```python
from build123d import *

# Parameters (mm, degrees)
F0_R      = 15.24
F0_R_2    = 11.43
F1_DEPTH  = 2.9972
F3_DEPTH  = 26.67
F4_R      = 15.24
F4_R_2    = 11.43
F5_DEPTH  = 2.54
F6_W      = 9.144
F6_H      = 6.35
F7_DEPTH  = 28.575
F8_W      = 1.27
F8_H      = 6.096
F9_DEPTH  = 2.54
F10_R     = 24.638
F10_R_2   = 15.24
F11_DEPTH = 3.81
F12_DEPTH = 11.43
F13_R     = 15.24
F13_R_2   = 11.43
F14_DEPTH = 20.955
F16_DEPTH = 3.4544
F17_R     = 15.24
F17_R_2   = 11.43
F18_DEPTH = 3.175
F19_DEPTH = 25.4
F20_R     = 1.5621
F21_DEPTH = 6.35


with BuildPart() as f1:
    # F0 (on Front) → F1 (new body)
    with BuildSketch(Plane.XZ):
        Circle(F0_R)
        Circle(F0_R_2, mode=Mode.SUBTRACT)
    extrude(amount=F1_DEPTH)

    # F2 (on face) → F3 (join)
    with BuildSketch(Plane.XZ.offset(2.9972)):
        with BuildLine():
            Line((15.24, 0), (12.7, 0))
            ThreePointArc((12.7, 0), (0, -12.7), (-12.7, 0))
            Line((-12.7, 0), (-15.24, 0))
            ThreePointArc((-15.24, 0), (0, -15.24), (15.24, 0))
        make_face()
    extrude(amount=F3_DEPTH)

    # F4 (on face) → F5 (join)
    with BuildSketch(Plane.XZ.offset(29.6672)):
        Circle(F4_R)
        Circle(F4_R_2, mode=Mode.SUBTRACT)
    extrude(amount=F5_DEPTH)

    # F6 (on Top) → F7 (cut)
    with BuildSketch(Plane.XY):
        Polygon((-13.335, -64.7192), (-13.335, -68.0212), (-4.572, -68.0212), (4.572, -68.0212), (13.335, -68.0212), (13.335, -64.7192), align=None)
        with Locations((0, -71.1962)):
            Rectangle(F6_W, F6_H)
    extrude(amount=F7_DEPTH, mode=Mode.SUBTRACT)

    # F8 (on face) → F9 (join)
    with BuildSketch(Plane.XY):
        with Locations((13.97, -15.0622)):
            Rectangle(F8_W, F8_H)
        with Locations((-13.97, -15.0622)):
            Rectangle(F8_W, F8_H)
    extrude(amount=F9_DEPTH)

    # F10 (on face) → F11 (join)
    with BuildSketch(Plane.XZ.offset(32.2072)):
        Circle(F10_R)
        Circle(F10_R_2, mode=Mode.SUBTRACT)
    extrude(amount=-F11_DEPTH)

    # F12 (add): a face of the model
    f12_faces = [f1.faces().sort_by_distance(p)[0] for p in [
        (-23.941132125, -32.2072, 0),
    ]]
    extrude(f12_faces, amount=F12_DEPTH)

    # F13 (on face) → F14 (join)
    with BuildSketch(Plane.XZ.offset(43.6372)):
        Circle(F13_R)
        Circle(F13_R_2, mode=Mode.SUBTRACT)
    extrude(amount=F14_DEPTH)

    # F15 (on face) → F16 (join)
    with BuildSketch(Plane.XZ.offset(64.5922)):
        with BuildLine():
            Line((13.335, 7.3780332745), (13.335, 0))
            ThreePointArc((13.335, 0), (0, -13.335), (-13.335, 0))
            Line((-13.335, 0), (-13.335, 7.3780332745))
            ThreePointArc((-13.335, 7.3780332745), (-3.81, -14.7560665491), (15.24, 0))
            ThreePointArc((15.24, 0), (14.7560665491, 3.81), (13.335, 7.3780332745))
        make_face()
    extrude(amount=F16_DEPTH)

    # F17 (on face) → F18 (join)
    with BuildSketch(Plane.XZ.offset(68.0466)):
        Circle(F17_R)
        Circle(F17_R_2, mode=Mode.SUBTRACT)
    extrude(amount=F18_DEPTH)

    # F6 (on Top) → F19 (cut)
    with BuildSketch(Plane.XY):
        Polygon((-13.335, -64.7192), (-13.335, -68.0212), (-4.572, -68.0212), (4.572, -68.0212), (13.335, -68.0212), (13.335, -64.7192), align=None)
        with Locations((0, -71.1962)):
            Rectangle(F6_W, F6_H)
    extrude(amount=F19_DEPTH, mode=Mode.SUBTRACT)

    # F20 (on face) → F21 (join)
    with BuildSketch(Plane.XZ.offset(43.6372)):
        with Locations((20.828, 0)):
            Circle(F20_R)
        with Locations((-20.828, 0)):
            Circle(F20_R)
    extrude(amount=F21_DEPTH)


solid = f1.part
```
The listing builds one solid part. Answer for the finished solid, in the listing's coordinates (mm). A direction names the side the tool comes from. Give positions to 0.01 mm unless a question says otherwise; leave off trailing zeros. Write each loop counter-clockwise with the first axis right and the second up, starting at its lowest first coordinate (ties: lowest second). Pieces come first, ordered by that corner, then holes. Notation, with made-up numbers: (-24.5, 79.5) -> (-18.5, 79.5) arc R28 ccw to (-18.5, 107.5) -> close; hole circle Ø4 at (-30.5, -36). An arc over 180 degrees is marked (long way). Use one line per item in the form item = value.
1) Each of these flat-tipped pins is pushed along its axis until it touches: P1, Ø14, axis at x = 3, z = 3.5, coming from the -Y side; P2, Ø3, axis at x = -15.5, y = -46, coming from the +Z side; P3, Ø12, axis at x = 14.5, y = -13.5, coming from the +Z side; P4, Ø18.5, axis at x = 0, z = 0, coming from the +Y side. Where does it stop, or does it pass through?
Result:
P1 = -71.22
P2 = 6.02
P3 = 2.54
P4 = through
2) For a pull along Z with two mould halves and no side action, classify faces 1 (the flat face through (-1, -29.667, 12)), 2 (the flat face through (-21, -49.987, 0)) as +Z half, -Z half, draft (parallel to the pull), parting line (faces both ways), or undercut.
Result:
face_1 = undercut
face_2 = draft
3) Straight lines are drawn through the part: probe 1 along Y at (x, z) = (6, -11); probe 2 along Z at (x, y) = (0, -0.7). For each, find the intervals that lie inside material, in ascending order.
Result:
probe_1 = -71.22 to -68.05, -64.59 to -29.67, -3 to 0
probe_2 = -15.24 to -11.43, 11.43 to 15.24
4) Section A-A on x = 0 is taken. Write down the section's boundary in (y, z) (3 decimals), plus the area to 3 significant figures.
Result:
outline = (-71.222, -15.24) -> (-43.637, -15.24) -> (-43.637, -24.638) -> (-28.397, -24.638) -> (-28.397, -15.24) -> (0, -15.24) -> (0, -11.43) -> (-2.997, -11.43) -> (-2.997, -12.7) -> (-29.667, -12.7) -> (-29.667, -11.43) -> (-64.592, -11.43) -> (-64.592, -13.335) -> (-68.047, -13.335) -> (-68.047, -11.43) -> (-71.222, -11.43) -> close; (-64.592, 11.43) -> (-29.667, 11.43) -> (-29.667, 15.24) -> (-28.397, 15.24) -> (-28.397, 24.638) -> (-43.637, 24.638) -> (-43.637, 15.24) -> (-64.592, 15.24) -> close; (-2.997, 11.43) -> (0, 11.43) -> (0, 15.24) -> (-2.997, 15.24) -> close
area = 662 mm²
5) Section D-D on y = -13.5 is taken. Write down the section's boundary in (x, z) (3 decimals), plus the area to 3 significant figures.
Result:
outline = (-15.24, 0) arc R15.24 ccw to (15.24, 0) -> (14.605, 0) -> (14.605, 2.54) -> (13.335, 2.54) -> (13.335, 0) -> (12.7, 0) arc R12.7 cw to (-12.7, 0) -> (-13.335, 0) -> (-13.335, 2.54) -> (-14.605, 2.54) -> (-14.605, 0) -> close
area = 118 mm²
6) Section C-C on x = -6 is taken. Count the separate pieces of the cut face and the enclosed holes in it, plus the area to 3 significant figures.
Result:
separate_pieces = 4
enclosed_holes = 0
area = 736 mm²
7) A tool of negligible diameter and unlimited length cuts with its end or side. For faces 3 (the flat face through (-4.572, -70, 12)), 4 (the flat face through (14.605, -15, 1)), 5 (the flat face through (13.335, -66, 4)), from which of +Z, -Z, +X, -X, +Y, -Y can it reach the whole face along a straight path? Write none if from no direction.
Result:
face_3 = +Z, -Y
face_4 = +Z, +X
face_5 = +Z
